Part model, mm, in its own coordinate system. A direction names the side the tool comes from. Round coordinates to 2 decimals unless told otherwise and drop trailing zeros. Write each loop counter-clockwise with the first axis right and the second up, starting at its lowest first coordinate (ties: lowest second). Pieces come first, ordered by that corner, then holes. Notation, with made-up numbers: M 43,-22 L 97,-22 A26 cw 97,1 Z; hole C -16.75,-15.5 d9. An arc over 180 degrees is marked long. Answer as a JSON object with one key per item and string values. Group by question number.
1. Drill centre lines: line 1 (X direction, y = 8.75, z = 3.5); line 2 (Z direction, x = 7, y = 22); line 3 (Y direction, x = 19.5, z = 30). Where is each one in solid material? Low to high. Write a range as from..to.
2. Band-saw the part on D-D, the plane x = 14.5. Write the cut outline in (y, z).
3. Which spindle directions (+Z, -Z, +X, -X, +Y, -Y) get a long thin tool onto all of the face, cutting with end or side? Do faces 5 (the face through (-42, 6, 17)), 6 (the face through (-42, 8, 7)), 7 (the face through (-1, 14, -34)). Say none if no direction does.
4. Drop flat-ended pins along their axis: pin 1 (1 mm diameter, centred on x = -41.5, y = 7.5, fed in from -Z); pin 2 (1 mm diameter, centred on x = -20, z = 4.5, fed in from +Y); pin 3 (1.6 mm diameter, centred on y = 11, z = 35.5, fed in from +X). Give the stop position or say it passes through.
5. Band-saw the part on C-C, the plane y = 14.25. Write the cut outline in (x, z).
6. Band-saw the part on A-A, the plane z = -30. Write the cut outline in (x, y), plus the area to 3 significant figures.
7. Band-saw the part on B-B, the plane z = -15.5. Write the cut outline in (x, y).
8. Two-plate mould, pull along Z, no slides. Class faces 1 (the face through (-41.93, 0.6, -0.48)), 2 (the face through (-42, 7, -33)), 3 (the face through (42, 6, -9)), 4 (the face through (41.9, 14.17, -35.43)): +Z half, -Z half, draft (parallel to the pull), parting line (faces both ways), or undercut.
from build123d import *

# Parameters (mm, degrees)
ESQUISSE1_W             = 85
ESQUISSE1_H             = 72
BOSS_EXTRU_1_DEPTH      = 26
COQUE1_T                = -2
ESQUISSE2_R             = 5
ESQUISSE2_W             = 10
ESQUISSE2_H             = 8
ENL_V_MAT_EXTRU_1_DEPTH = 2
ESQUISSE3_W             = 15
ESQUISSE3_H             = 5
ENL_V_MAT_EXTRU_2_DEPTH = 2
ESQUISSE4_W             = 7
ESQUISSE4_H             = 22
ENL_V_MAT_EXTRU_3_DEPTH = 2
ESQUISSE5_W             = 20
ESQUISSE5_H             = 5
ENL_V_MAT_EXTRU_4_DEPTH = 2
ESQUISSE6_W             = 15
ESQUISSE6_H             = 5
ENL_V_MAT_EXTRU_5_DEPTH = 2
ENL_V_MAT_EXTRU_7_DEPTH = 2
CONG_1_R                = 2


with BuildPart() as part:
    # Esquisse1 → Boss.-Extru.1 (new body)
    with BuildSketch(Plane(origin=(0, 0, 0), x_dir=(1, 0, 0), z_dir=(0, 1, 0))):
        Rectangle(ESQUISSE1_W, ESQUISSE1_H)
    extrude(amount=BOSS_EXTRU_1_DEPTH)

    # Coque1
    coque1_openings = [part.faces().sort_by_distance(p)[0] for p in [
        (0, 26, 0),
    ]]
    offset(amount=COQUE1_T, openings=coque1_openings, kind=Kind.INTERSECTION)

    # Esquisse2 → Enlèv. mat.-Extru.1 (cut)
    with BuildSketch(Plane(origin=(42.5, 0, 0), x_dir=(0, 0, -1), z_dir=(1, 0, 0))):
        with Locations((27, 18)):
            Circle(ESQUISSE2_R)
        with Locations((27, 22)):
            Rectangle(ESQUISSE2_W, ESQUISSE2_H)
    extrude(amount=-ENL_V_MAT_EXTRU_1_DEPTH, mode=Mode.SUBTRACT)

    # Esquisse3 → Enlèv. mat.-Extru.2 (cut)
    with BuildSketch(Plane(origin=(42.5, 0, 0), x_dir=(0, 0, -1), z_dir=(1, 0, 0))):
        with Locations((9.5, 8.5)):
            Rectangle(ESQUISSE3_W, ESQUISSE3_H)
        with Locations((-11.5, 8.5)):
            Rectangle(ESQUISSE3_W, ESQUISSE3_H)
    extrude(amount=-ENL_V_MAT_EXTRU_2_DEPTH, mode=Mode.SUBTRACT)

    # Esquisse4 → Enlèv. mat.-Extru.3 (cut)
    with BuildSketch(Plane.XY.offset(36)):
        with Locations((27, 15)):
            Rectangle(ESQUISSE4_W, ESQUISSE4_H)
    extrude(amount=-ENL_V_MAT_EXTRU_3_DEPTH, mode=Mode.SUBTRACT)

    # Esquisse5 → Enlèv. mat.-Extru.4 (cut)
    with BuildSketch(Plane.ZY.offset(42.5)):
        with Locations((17, 8.5)):
            Rectangle(ESQUISSE5_W, ESQUISSE5_H)
    extrude(amount=-ENL_V_MAT_EXTRU_4_DEPTH, mode=Mode.SUBTRACT)

    # Esquisse6 → Enlèv. mat.-Extru.5 (cut)
    with BuildSketch(Plane.ZY.offset(42.5)):
        with Locations((-11.5, 8.5)):
            Rectangle(ESQUISSE6_W, ESQUISSE6_H)
    extrude(amount=-ENL_V_MAT_EXTRU_5_DEPTH, mode=Mode.SUBTRACT)

    # Esquisse8 → Enlèv. mat.-Extru.7 (cut)
    with BuildSketch(Plane.ZY.offset(42.5)):
        with BuildLine():
            Line((-31.5, 10), (-22.5, 10))
            ThreePointArc((-22.5, 10), (-21.439339828, 9.560660172), (-21, 8.5))
            Line((-21, 8.5), (-21, 5.5))
            ThreePointArc((-21, 5.5), (-21.439339828, 4.439339828), (-22.5, 4))
            Line((-22.5, 4), (-31.5, 4))
            ThreePointArc((-31.5, 4), (-32.560660172, 4.439339828), (-33, 5.5))
            Line((-33, 5.5), (-33, 8.5))
            ThreePointArc((-33, 8.5), (-32.560660172, 9.560660172), (-31.5, 10))
        make_face()
    extrude(amount=-ENL_V_MAT_EXTRU_7_DEPTH, mode=Mode.SUBTRACT)

    # Congé1
    cong_1_edges = [part.edges().sort_by_distance(p)[0] for p in [
        (0, 0, -36),
        (42.5, 0, 0),
        (0, 0, 36),
        (-42.5, 0, 0),
        (-42.5, 13, -36),
        (42.5, 13, -36),
        (42.5, 13, 36),
        (-42.5, 13, 36),
    ]]
    fillet(cong_1_edges, radius=CONG_1_R)


solid = part.part
Worked answers:
{
 "1": {"line 1": "x = -42.5..-40.5, 40.5..42.5", "line 2": "z = -36..-34, 34..36", "line 3": "y = 0..2"},
 "2": {"outline": "M 0,-34 A2 ccw 2,-36 L 26,-36 L 26,-34 L 2,-34 L 2,34 L 26,34 L 26,36 L 2,36 A2 ccw 0,34 Z"},
 "3": {"face 5": "-X", "face 6": "+X, -X", "face 7": "+Y"},
 "4": {"pin 1": "stops at z = -35.94", "pin 2": "stops at y = 2", "pin 3": "stops at x = 42.37"},
 "5": {"outline": "M -42.5,-34 A2 ccw -40.5,-36 L 40.5,-36 A2 ccw 42.5,-34 L 42.5,-30.31 L 40.5,-30.31 L 40.5,-34 L -40.5,-34 L -40.5,34 L 23.5,34 L 23.5,36 L -40.5,36 A2 ccw -42.5,34 Z; M 30.5,34 L 40.5,34 L 40.5,-23.69 L 42.5,-23.69 L 42.5,34 A2 ccw 40.5,36 L 30.5,36 Z"},
 "6": {"outline": "M -42.5,2 A2 ccw -40.5,0 L 40.5,0 A2 ccw 42.5,2 L 42.5,14 L 40.5,14 L 40.5,2 L -40.5,2 L -40.5,4 L -42.5,4 Z; M -42.5,10 L -40.5,10 L -40.5,26 L -42.5,26 Z", "area": "228 mm^2"},
 "7": {"outline": "M -42.5,2 A2 ccw -40.5,0 L 40.5,0 A2 ccw 42.5,2 L 42.5,6 L 40.5,6 L 40.5,2 L -40.5,2 L -40.5,6 L -42.5,6 Z; M -42.5,11 L -40.5,11 L -40.5,26 L -42.5,26 Z; M 40.5,11 L 42.5,11 L 42.5,26 L 40.5,26 Z"},
 "8": {"face 1": "draft", "face 2": "undercut", "face 3": "undercut", "face 4": "-Z half"}
}
